Design review of the part built by this model. Coordinates are the model's own, in mm. Coordinates: 2 decimals unless noted, no trailing zeros. Write each loop counter-clockwise with the first axis right and the second up, starting at its lowest first coordinate (ties: lowest second). Pieces come first, ordered by that corner, then holes. Notation, with made-up numbers: (58, 24) - (113, 24) arc R26 ccw to (113, 48) - close; hole circle Ø5 at (21.25, 23). An arc over 180 degrees is marked (long way). One line per item, written item: value.
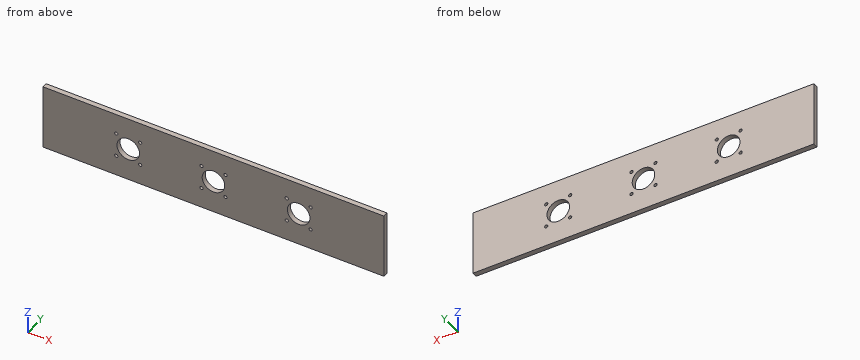
from build123d import *

# Parameters (mm, degrees)
F0_W     = 431.8
F0_H     = 82.55
F1_DEPTH = 6.35
F3_DEPTH = 6.35
F5_DEPTH = 6.35


with BuildPart() as f1:
    # F0 (on Front) → F1 (new body)
    with BuildSketch(Plane.XZ):
        Rectangle(F0_W, F0_H)
    extrude(amount=F1_DEPTH)

    # F2 (on face) → F3 (cut, through all)
    with BuildSketch(Plane.XZ.offset(6.35)):
        with BuildLine():
            Line((-122.2375, 0), (-93.6625, 0))
            ThreePointArc((-93.6625, 0), (-107.95, 14.2875), (-122.2375, 0))
        make_face()
        with BuildLine():
            ThreePointArc((-122.2375, 0), (-107.95, -14.2875), (-93.6625, 0))
            Line((-93.6625, 0), (-122.2375, 0))
        make_face()
        with BuildLine():
            ThreePointArc((-14.2875, 0), (0, -14.2875), (14.2875, 0))
            Line((14.2875, 0), (-14.2875, 0))
        make_face()
        with BuildLine():
            Line((-14.2875, 0), (14.2875, 0))
            ThreePointArc((14.2875, 0), (0, 14.2875), (-14.2875, 0))
        make_face()
        with BuildLine():
            ThreePointArc((93.6625, 0), (107.95, -14.2875), (122.2375, 0))
            Line((122.2375, 0), (93.6625, 0))
        make_face()
        with BuildLine():
            Line((93.6625, 0), (122.2375, 0))
            ThreePointArc((122.2375, 0), (107.95, 14.2875), (93.6625, 0))
        make_face()
    extrude(amount=-F3_DEPTH, mode=Mode.SUBTRACT)

    # F4 (on face) → F5 (cut, through all)
    with BuildSketch(Plane.XZ.offset(6.35)):
        with BuildLine():
            ThreePointArc((-90.77325, -15.15745), (-91.3646892767, -13.7295892768), (-92.79255, -13.13815))
            Line((-92.79255, -13.13815), (-92.79255, -15.15745))
            Line((-92.79255, -15.15745), (-94.81185, -15.15745))
            ThreePointArc((-94.81185, -15.15745), (-92.79255, -17.17675), (-90.77325, -15.15745))
        make_face()
        with BuildLine():
            Line((-92.79255, -15.15745), (-92.79255, -13.13815))
            ThreePointArc((-92.79255, -13.13815), (-94.2204107232, -13.7295892767), (-94.81185, -15.15745))
            Line((-94.81185, -15.15745), (-92.79255, -15.15745))
        make_face()
        with BuildLine():
            ThreePointArc((-90.77325, 15.15745), (-92.79255, 17.17675), (-94.81185, 15.15745))
            Line((-94.81185, 15.15745), (-92.79255, 15.15745))
            Line((-92.79255, 15.15745), (-92.79255, 13.13815))
            ThreePointArc((-92.79255, 13.13815), (-91.3646892767, 13.7295892768), (-90.77325, 15.15745))
        make_face()
        with BuildLine():
            Line((-92.79255, 15.15745), (-94.81185, 15.15745))
            ThreePointArc((-94.81185, 15.15745), (-94.2204107232, 13.7295892767), (-92.79255, 13.13815))
            Line((-92.79255, 13.13815), (-92.79255, 15.15745))
        make_face()
        with BuildLine():
            ThreePointArc((-123.10745, -13.13815), (-124.5353107233, -16.5853107232), (-121.08815, -15.15745))
            Line((-121.08815, -15.15745), (-123.10745, -15.15745))
            Line((-123.10745, -15.15745), (-123.10745, -13.13815))
        make_face()
        with BuildLine():
            Line((-123.10745, -15.15745), (-121.08815, -15.15745))
            ThreePointArc((-121.08815, -15.15745), (-121.6795892767, -13.7295892768), (-123.10745, -13.13815))
            Line((-123.10745, -13.13815), (-123.10745, -15.15745))
        make_face()
        with BuildLine():
            ThreePointArc((-121.08815, 15.15745), (-124.5353107233, 16.5853107232), (-123.10745, 13.13815))
            ThreePointArc((-123.10745, 13.13815), (-121.6795892767, 13.7295892768), (-121.08815, 15.15745))
        make_face()
        with BuildLine():
            ThreePointArc((125.12675, -15.15745), (124.5353107233, -13.7295892768), (123.10745, -13.13815))
            Line((123.10745, -13.13815), (123.10745, -15.15745))
            Line((123.10745, -15.15745), (121.08815, -15.15745))
            ThreePointArc((121.08815, -15.15745), (123.10745, -17.17675), (125.12675, -15.15745))
        make_face()
        with BuildLine():
            Line((123.10745, -15.15745), (123.10745, -13.13815))
            ThreePointArc((123.10745, -13.13815), (121.6795892768, -13.7295892767), (121.08815, -15.15745))
            Line((121.08815, -15.15745), (123.10745, -15.15745))
        make_face()
        with BuildLine():
            ThreePointArc((125.12675, 15.15745), (123.10745, 17.17675), (121.08815, 15.15745))
            Line((121.08815, 15.15745), (123.10745, 15.15745))
            Line((123.10745, 15.15745), (123.10745, 13.13815))
            ThreePointArc((123.10745, 13.13815), (124.5353107233, 13.7295892768), (125.12675, 15.15745))
        make_face()
        with BuildLine():
            Line((123.10745, 15.15745), (121.08815, 15.15745))
            ThreePointArc((121.08815, 15.15745), (121.6795892768, 13.7295892767), (123.10745, 13.13815))
            Line((123.10745, 13.13815), (123.10745, 15.15745))
        make_face()
        with BuildLine():
            ThreePointArc((94.81185, 15.15745), (91.3646892767, 16.5853107232), (92.79255, 13.13815))
            ThreePointArc((92.79255, 13.13815), (94.2204107233, 13.7295892768), (94.81185, 15.15745))
        make_face()
        with BuildLine():
            ThreePointArc((92.79255, -13.13815), (91.3646892767, -16.5853107232), (94.81185, -15.15745))
            Line((94.81185, -15.15745), (92.79255, -15.15745))
            Line((92.79255, -15.15745), (92.79255, -13.13815))
        make_face()
        with BuildLine():
            Line((92.79255, -15.15745), (94.81185, -15.15745))
            ThreePointArc((94.81185, -15.15745), (94.2204107233, -13.7295892768), (92.79255, -13.13815))
            Line((92.79255, -13.13815), (92.79255, -15.15745))
        make_face()
        with BuildLine():
            ThreePointArc((-15.15745, -13.13815), (-16.5853107233, -16.5853107232), (-13.13815, -15.15745))
            Line((-13.13815, -15.15745), (-15.15745, -15.15745))
            Line((-15.15745, -15.15745), (-15.15745, -13.13815))
        make_face()
        with BuildLine():
            Line((-15.15745, -15.15745), (-13.13815, -15.15745))
            ThreePointArc((-13.13815, -15.15745), (-13.7295892767, -13.7295892768), (-15.15745, -13.13815))
            Line((-15.15745, -13.13815), (-15.15745, -15.15745))
        make_face()
        with BuildLine():
            ThreePointArc((17.17675, -15.15745), (16.5853107233, -13.7295892768), (15.15745, -13.13815))
            Line((15.15745, -13.13815), (15.15745, -15.15745))
            Line((15.15745, -15.15745), (13.13815, -15.15745))
            ThreePointArc((13.13815, -15.15745), (15.15745, -17.17675), (17.17675, -15.15745))
        make_face()
        with BuildLine():
            Line((15.15745, -15.15745), (15.15745, -13.13815))
            ThreePointArc((15.15745, -13.13815), (13.7295892768, -13.7295892767), (13.13815, -15.15745))
            Line((13.13815, -15.15745), (15.15745, -15.15745))
        make_face()
        with BuildLine():
            ThreePointArc((17.17675, 15.15745), (15.15745, 17.17675), (13.13815, 15.15745))
            Line((13.13815, 15.15745), (15.15745, 15.15745))
            Line((15.15745, 15.15745), (15.15745, 13.13815))
            ThreePointArc((15.15745, 13.13815), (16.5853107233, 13.7295892768), (17.17675, 15.15745))
        make_face()
        with BuildLine():
            Line((15.15745, 15.15745), (13.13815, 15.15745))
            ThreePointArc((13.13815, 15.15745), (13.7295892768, 13.7295892767), (15.15745, 13.13815))
            Line((15.15745, 13.13815), (15.15745, 15.15745))
        make_face()
        with BuildLine():
            ThreePointArc((-13.13815, 15.15745), (-16.5853107233, 16.5853107232), (-15.15745, 13.13815))
            ThreePointArc((-15.15745, 13.13815), (-13.7295892767, 13.7295892768), (-13.13815, 15.15745))
        make_face()
    extrude(amount=-F5_DEPTH, mode=Mode.SUBTRACT)


solid = f1.part
1. Consider section B-B, the plane z = -4. Write out the cut boundary in (x, y), then the cut area to 3 significant figures.
Answer block:
outline: (-215.9, -6.35) - (-121.67, -6.35) - (-121.67, 0) - (-215.9, 0) - close; (-94.23, -6.35) - (-13.72, -6.35) - (-13.72, 0) - (-94.23, 0) - close; (13.72, -6.35) - (94.23, -6.35) - (94.23, 0) - (13.72, 0) - close; (121.67, -6.35) - (215.9, -6.35) - (215.9, 0) - (121.67, 0) - close
area: 2,220 mm^2
2. Consider section C-C, the plane y = -4. Give the number of separate pieces and of enclosed holes in the cut face, then the cut area to 3 significant figures.
Answer block:
separate pieces: 1
enclosed holes: 15
area: 33,600 mm^2
3. Wall thickness on line 1 along X through (y, z) = (-0.25, -0.5); line 2 along Z through (x, y) = (-107.95, -2) (1 decimal); line 3 along X through (y, z) = (-3, -10.5): over which ranges is each line inside the solid? List them lowest first.
Answer block:
line 1: x = -215.9 to -122.23, -93.67 to -14.28, 14.28 to 93.67, 122.23 to 215.9
line 2: z = -41.3 to -14.3, 14.3 to 41.3
line 3: x = -215.9 to -117.64, -98.26 to -9.69, 9.69 to 98.26, 117.64 to 215.9
4. Insertion check: pin 1 Ø3.5 at (x, z) = (92.79, 15.16) entering from -Y; pin 2 Ø10 at (x, z) = (-30.5, -6.5) entering from +Y. Each pin has a flat end and moves straight along its axis. Give the tip position at first contact, or say it passes through.
Answer block:
pin 1: passes through
pin 2: stops at y = 0
